```python
from build123d import *

# Parameters (mm, degrees)
EXTRUDE_1_DEPTH     = 50
SKETCH_3_W          = 3
SKETCH_3_H          = 11.5
CUT_EXTRUDE_1_DEPTH = 1.5
FILLET_1_R          = 1.5


with BuildPart() as part:
    # 草图1 → 凸台-拉伸1 (new body)
    with BuildSketch(Plane.XY):
        with BuildLine():
            Line((-40.582688737, 29.861069553), (147.917311263, 29.861069553))
            Line((147.917311263, 29.861069553), (147.917311263, 31.361069553))
            Line((147.917311263, 31.361069553), (-42.082688737, 31.361069553))
            ThreePointArc((-42.082688737, 31.361069553), (-43.143348909, 30.921729725), (-43.582688737, 29.861069553))
            Line((-43.582688737, 29.861069553), (-43.582688737, -236.138930447))
            ThreePointArc((-43.582688737, -236.138930447), (-43.143348909, -237.199590619), (-42.082688737, -237.638930447))
            Line((-42.082688737, -237.638930447), (-15.082688737, -237.638930447))
            Line((-15.082688737, -237.638930447), (-13.582688737, -237.638930447))
            Line((-13.582688737, -237.638930447), (-13.582688737, -236.138930447))
            Line((-13.582688737, -236.138930447), (-13.582688737, -226.138930447))
            Line((-13.582688737, -226.138930447), (-15.082688737, -226.138930447))
            Line((-15.082688737, -226.138930447), (-15.082688737, -234.638930447))
            Line((-15.082688737, -234.638930447), (-15.082688737, -236.138930447))
            Line((-15.082688737, -236.138930447), (-16.582688737, -236.138930447))
            Line((-16.582688737, -236.138930447), (-40.582688737, -236.138930447))
            ThreePointArc((-40.582688737, -236.138930447), (-41.643348909, -235.699590619), (-42.082688737, -234.638930447))
            Line((-42.082688737, -234.638930447), (-42.082688737, -226.138930447))
            Line((-42.082688737, -226.138930447), (-42.082688737, -50.138930447))
            Line((-42.082688737, -50.138930447), (-42.082688737, 28.361069553))
            ThreePointArc((-42.082688737, 28.361069553), (-41.643348909, 29.421729725), (-40.582688737, 29.861069553))
        make_face()
    extrude(amount=EXTRUDE_1_DEPTH)

    # 草图3 → 切除-拉伸1 (cut)
    with BuildSketch(Plane(origin=(-13.582688737, 0, 0), x_dir=(0, 0, -1), z_dir=(1, 0, 0))):
        with Locations((-48.5, -231.888930447)):
            Rectangle(SKETCH_3_W, SKETCH_3_H)
        with Locations((-1.5, -231.888930447)):
            Rectangle(SKETCH_3_W, SKETCH_3_H)
    extrude(amount=-CUT_EXTRUDE_1_DEPTH, mode=Mode.SUBTRACT)

    # 圆角1
    fillet_1_edges = [part.edges().sort_by_distance(p)[0] for p in [
        (-13.582688737, -237.638930447, 25),
    ]]
    fillet(fillet_1_edges, radius=FILLET_1_R)


solid = part.part
```
Design review of the part built by this model. Coordinates are the model's own, in mm. A direction names the side the tool comes from. Give positions to 0.01 mm unless a question says otherwise; leave off trailing zeros. Order: outer loops, then holes, each group sorted by start corner. A loop starts at its lowest first (then second) coordinate and runs counter-clockwise, first axis right, second up. Notation, with made-up numbers: (18.25, 85.5) - (27.25, 85.5) arc R12 cw to (27.25, 94.5) - close; hole circle Ø10 at (-26, 69). An arc over 180 degrees is marked (long way). Use a Markdown table: item, result. Add a question column.
(1) Add section B-B on x = 132. Give the boundary of the cut face in (y, z), then the cut area to 3 significant figures.
(2) Clearance check with flat-ended pins moving along their axes: P1, Ø1.7, axis at x = -14, y = -229, coming from the -Z side; P2, Ø3, axis at x = 124, z = 7.5, coming from the -Y side; P3, Ø11, axis at y = -229, z = 21.5, coming from the +X side. State where each tip first meets the part, or that it passes through.
(3) Add section A-A on z = 25.5. Give the boundary of the cut face in (x, y), then the cut area to 3 significant figures.
(4) Mouldability with a two-part tool opening along X and no side actions: class faces 1 (the face through (54, 31.361, 25)), 2 (the face through (-13.583, -231, 25)), 3 (the face through (-15.083, -231, 25)), 4 (the face through (-43.583, -101, 25)) as +X half, -X half, draft (parallel to the pull), parting line (faces both ways), or undercut.
(5) Wall thickness on probe 1 along Y at (x, z) = (-20, 5.5); probe 2 along Y at (x, z) = (62, 23.5); probe 3 along X at (y, z) = (9.5, 25): over which ranges is each line inside the solid? List them lowest first. Write a range as [from, to].
(6) Add section C-C on y = -122. Give the boundary of the cut face in (x, z).
(7) Machinability: for faces 5 (the face through (-29, -237.639, 25)), 6 (the face through (-28, -236.139, 25)), which of the approach directions +Z, -Z, +X, -X, +Y, -Y give a long, thin tool a straight path to every point of the face, cutting with its end or side? Answer none if there is none.
Report:
| question | item | result |
|---|---|---|
| 1 | outline | (29.86, 0) - (31.36, 0) - (31.36, 50) - (29.86, 50) - close |
| 1 | area | 75.0 mm² |
| 2 | P1 | stops at z = 3 |
| 2 | P2 | stops at y = 29.86 |
| 2 | P3 | stops at x = -13.58 |
| 3 | outline | (-43.58, -236.14) arc R1.5 ccw to (-42.08, -237.64) - (-15.08, -237.64) arc R1.5 ccw to (-13.58, -236.14) - (-13.58, -226.14) - (-15.08, -226.14) - (-15.08, -236.14) - (-40.58, -236.14) arc R1.5 cw to (-42.08, -234.64) - (-42.08, 28.36) arc R1.5 cw to (-40.58, 29.86) - (147.92, 29.86) - (147.92, 31.36) - (-42.08, 31.36) arc R1.5 ccw to (-43.58, 29.86) - close |
| 3 | area | 746 mm² |
| 4 | face 1 | draft |
| 4 | face 2 | +X half |
| 4 | face 3 | undercut |
| 4 | face 4 | -X half |
| 5 | probe 1 | y = [-237.64, -236.14], [29.86, 31.36] |
| 5 | probe 2 | y = [29.86, 31.36] |
| 5 | probe 3 | x = [-43.58, -42.08] |
| 6 | outline | (-43.58, 0) - (-42.08, 0) - (-42.08, 50) - (-43.58, 50) - close |
| 7 | face 5 | +Z, -Z, +X, -X, -Y |
| 7 | face 6 | +Z, -Z |
